from build123d import *

# Parameters (mm, degrees)
SKETCH_R  = 4.5
PAD_DEPTH = 12


with BuildPart() as part:
    # Sketch → Pad (new body)
    with BuildSketch(Plane.XY):
        with BuildLine():
            Line((0, -2), (0, -23.171573))
            ThreePointArc((0, -23.171573), (1.234633, -25.019332), (3.414214, -24.585786))
            Line((3.414214, -24.585786), (24.585786, -3.414214))
            ThreePointArc((24.585786, -3.414214), (25.019332, -1.234633), (23.171573, 0))
            Line((23.171573, 0), (2, 0))
            ThreePointArc((2, 0), (0.585786, -0.585786), (0, -2))
        make_face()
        with Locations((9, -9)):
            Circle(SKETCH_R, mode=Mode.SUBTRACT)
    extrude(amount=PAD_DEPTH)


solid = part.part
Can you work these out from the model? Positions are in its coordinate system, mm. Give positions to 0.01 mm unless a question says otherwise; leave off trailing zeros. Loops run counter-clockwise (first coordinate to the right, second up) from the corner with the lowest first, then second, coordinate; pieces in that order, holes last. Notation, with made-up numbers: (-29.5, 53) -> (29.5, 53) arc R12 ccw to (29.5, 73) -> close; hole circle Ø4 at (67.25, -23.75). An arc over 180 degrees is marked (long way). Write item = value, one per line.
1) Suppose I cut it at B-B on x = 9. Write out the boundary of the cut face in (y, z).
Check result:
outline = (-19, 0) -> (-13.5, 0) -> (-13.5, 12) -> (-19, 12) -> close; (-4.5, 0) -> (0, 0) -> (0, 12) -> (-4.5, 12) -> close
2) Suppose I cut it at A-A on y = -9. Write out the boundary of the cut face in (x, z).
Check result:
outline = (0, 0) -> (4.5, 0) -> (4.5, 12) -> (0, 12) -> close; (13.5, 0) -> (19, 0) -> (19, 12) -> (13.5, 12) -> close
3) Suppose I cut it at C-C on z = 1. Write out the boundary of the cut face in (x, y).
Check result:
outline = (0, -23.17) arc R2 ccw to (3.41, -24.59) -> (24.59, -3.41) arc R2 ccw to (23.17, 0) -> (2, 0) arc R2 ccw to (0, -2) -> close; hole circle Ø9 at (9, -9)
4) Suppose I cut it at D-D on x = 20. Write out the boundary of the cut face in (y, z), then the cut area to 3 significant figures.
Check result:
outline = (-8, 0) -> (0, 0) -> (0, 12) -> (-8, 12) -> close
area = 96.0 mm2
5) Will these pins go through, and if not, where does the flat tip stop? pin 1 (2 mm diameter, centred on x = 21.5, z = 4.5, fed in from -Y); pin 2 (1.5 mm diameter, centred on x = 20, z = 5, fed in from -Y); pin 3 (8 mm diameter, centred on x = 12, y = -4, fed in from -Z).
Check result:
pin_1 = -7.5
pin_2 = -8.75
pin_3 = 0
6) Thinking about a two-plate mould opening in Y: for faces 1 (the cylindrical face through (13.292, -7.648, 5.916)), 2 (the cylindrical face through (1.204, -25.006, 5.916)), 3 (the flat face through (12.4, -12.4, 12)), which applies, released by +Y, released by -Y, zero draft, split by the parting line, or undercut?
Check result:
face_1 = undercut
face_2 = released by -Y
face_3 = zero draft
7) I need wall thicknesses on L1, parallel to X at y = -16, z = 11.5; L2, parallel to X at y = -7, z = 11; L3, parallel to Y at x = 9, z = 3.5. Which ranges of each line are inside material? Lowest first, please. Write a range as from..to.
Check result:
L1 = 0..12
L2 = 0..4.97, 13.03..21
L3 = -19..-13.5, -4.5..0
